Check sheet for the modelled part. Datum: model origin and axes. Units: mm. Round coordinates to 2 decimals unless told otherwise and drop trailing zeros. Loops run counter-clockwise (first coordinate to the right, second up) from the corner with the lowest first, then second, coordinate; pieces in that order, holes last. Notation, with made-up numbers: (38, -21) -> (90, -21) arc R28 cw to (90, 11) -> close; hole circle Ø5 at (-16, 75). An arc over 180 degrees is marked (long way). Return JSON: item names as keys, results as strings.
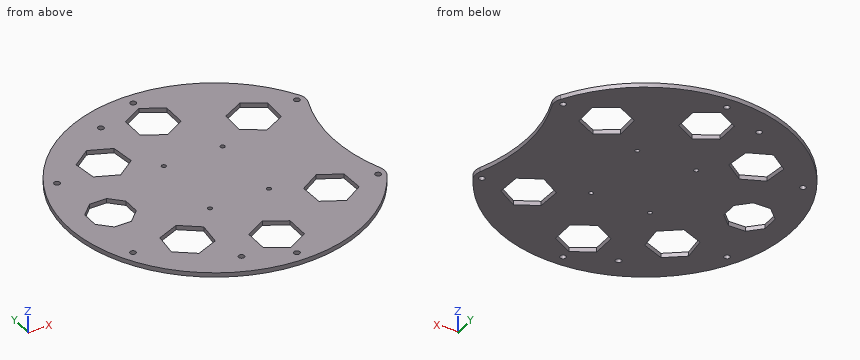
from build123d import *

# Parameters (mm, degrees)
CROQUIS1_R              = 100
SALIENTE_EXTRUIR1_DEPTH = 3
CROQUIS3_R              = 110
CORTAR_EXTRUIR1_DEPTH   = 3
REDONDEO1_R             = 10
CROQUIS4_R              = 1.5
CORTAR_EXTRUIR2_DEPTH   = 10
CORTAR_EXTRUIR3_DEPTH   = 10
CROQUIS6_R              = 2
CORTAR_EXTRUIR4_DEPTH   = 142.453172607


with BuildPart() as part:
    # Croquis1 → Saliente-Extruir1 (new body)
    with BuildSketch(Plane.XY):
        Circle(CROQUIS1_R)
    extrude(amount=SALIENTE_EXTRUIR1_DEPTH)

    # Croquis3 → Cortar-Extruir1 (cut)
    with BuildSketch(Plane.XY.offset(3)):
        with Locations((190, 0)):
            Circle(CROQUIS3_R)
    extrude(amount=-CORTAR_EXTRUIR1_DEPTH, mode=Mode.SUBTRACT)

    # Redondeo1
    redondeo1_edges = [part.edges().sort_by_distance(p)[0] for p in [
        (89.473684211, -44.659375654, 1.5),
        (89.473684211, 44.659375654, 1.5),
    ]]
    fillet(redondeo1_edges, radius=REDONDEO1_R)

    # Croquis4 → Cortar-Extruir2 (cut)
    with BuildSketch(Plane.XY.offset(3)):
        with Locations((-19.1, -26)):
            Circle(CROQUIS4_R)
        with Locations((20.9, -26)):
            Circle(CROQUIS4_R)
        with Locations((20.9, 26)):
            Circle(CROQUIS4_R)
        with Locations((-19.1, 26)):
            Circle(CROQUIS4_R)
    extrude(amount=-CORTAR_EXTRUIR2_DEPTH, mode=Mode.SUBTRACT)

    # Croquis5 → Cortar-Extruir3 (cut)
    with BuildSketch(Plane.XY.offset(3)):
        Polygon((66.297522474, -35.184824102), (66.874281495, -51.340339642), (53.171574136, -59.917585376), (38.892107757, -52.339315569), (38.315348736, -36.183800029), (52.018056095, -27.606554296), align=None)
        Polygon((14, 61.199128534), (14, 77.364936071), (0, 85.44783984), (-14, 77.364936071), (-14, 61.199128534), (0, 53.116224765), align=None)
        Polygon((-34.205975888, 56.833392886), (-49.063072127, 63.205207751), (-62.009773788, 53.524492414), (-60.099379209, 37.471962211), (-45.24228297, 31.100147347), (-32.295581309, 40.780862684), align=None)
        Polygon((66.874281495, 51.340339642), (53.171574136, 59.917585376), (38.892107757, 52.339315569), (38.315348736, 36.183800029), (52.018056095, 27.606554296), (66.297522474, 35.184824102), align=None)
        Polygon((-57, 5.798989873), (-65.201010127, 14), (-76.798989873, 14), (-85, 5.798989873), (-85, -5.798989873), (-76.798989873, -14), (-65.201010127, -14), (-57, -5.798989873), align=None)
        Polygon((0, -53.116224765), (14, -61.199128534), (14, -77.364936071), (0, -85.44783984), (-14, -77.364936071), (-14, -61.199128534), align=None)
        Polygon((-32.295581309, -40.780862684), (-34.205975888, -56.833392886), (-49.063072127, -63.205207751), (-62.009773788, -53.524492414), (-60.099379209, -37.471962211), (-45.24228297, -31.100147347), align=None)
    extrude(amount=-CORTAR_EXTRUIR3_DEPTH, mode=Mode.SUBTRACT)

    # Croquis6 → Cortar-Extruir4 (cut, through all)
    with BuildSketch(Plane.XY.offset(3)):
        with Locations((0, 92)):
            Circle(CROQUIS6_R)
        with Locations((83.182013697, 45.66031863)):
            Circle(CROQUIS6_R)
        with Locations((83.182013697, -45.66031863)):
            Circle(CROQUIS6_R)
        with Locations((0, -92)):
            Circle(CROQUIS6_R)
        with Locations((-81.512332571, -42.658406426)):
            Circle(CROQUIS6_R)
        with Locations((-81.512332571, 42.658406426)):
            Circle(CROQUIS6_R)
        with Locations(Location((-29.6, -78.7, 0), (0, 0, 180))):
            Circle(CROQUIS6_R)
        with Locations((-29.6, 79.3)):
            Circle(CROQUIS6_R)
    extrude(amount=-CORTAR_EXTRUIR4_DEPTH, mode=Mode.SUBTRACT)


solid = part.part
Q1. Section check A-A (x = 47). Record the boundary of the cut face in (y, z).
Results list:
{"outline": "(-88.27, 0) -> (-56.64, 0) -> (-56.64, 3) -> (-88.27, 3) -> close; (-30.75, 0) -> (30.75, 0) -> (30.75, 3) -> (-30.75, 3) -> close; (56.64, 0) -> (88.27, 0) -> (88.27, 3) -> (56.64, 3) -> close"}
Q2. Section check D-D (y = -69). Record the boundary of the cut face in (x, z), then the cut area to 3 significant figures.
Results list:
{"outline": "(-72.38, 0) -> (-14, 0) -> (-14, 3) -> (-72.38, 3) -> close; (14, 0) -> (72.38, 0) -> (72.38, 3) -> (14, 3) -> close", "area": "350 mm^2"}
Q3. Material ranges on line 1 (X direction, y = -35, z = 1.05); line 2 (Y direction, x = 62, z = 1.35); line 3 (X direction, y = -26.5, z = 2.8), recorded low to high.
Results list:
{"line 1": "-93.67 to -54.34, -40.03 to 40.21, 65.95 to 85.72", "line 2": "-78.46 to -54.39, -32.9 to 32.9, 54.39 to 78.46", "line 3": "-96.42 to -20.51, -17.69 to 19.49, 22.31 to 83.24"}
Q4. Section check B-B (y = 1). Record the boundary of the cut face in (x, z) (3 decimals).
Results list:
{"outline": "(-99.995, 0) -> (-85, 0) -> (-85, 3) -> (-99.995, 3) -> close; (-57, 0) -> (80.005, 0) -> (80.005, 3) -> (-57, 3) -> close"}
Q5. Go/stop test with flat-tipped pins: pin 1 (1 mm diameter, centred on y = 79, z = 2, fed in from -X); pin 2 (1.5 mm diameter, centred on y = -71.5, z = 1, fed in from -X); pin 3 (2.5 mm diameter, centred on x = 0, y = 92, fed in from +Z). Record where each tip stops, or that it passes through.
Results list:
{"pin 1": "x = -61.95", "pin 2": "x = -70.67", "pin 3": "through"}
Q6. Section check C-C (x = 7). Record the boundary of the cut face in (y, z).
Results list:
{"outline": "(-99.75, 0) -> (-81.41, 0) -> (-81.41, 3) -> (-99.75, 3) -> close; (-57.16, 0) -> (57.16, 0) -> (57.16, 3) -> (-57.16, 3) -> close; (81.41, 0) -> (99.75, 0) -> (99.75, 3) -> (81.41, 3) -> close"}
